```python
from build123d import *

# Parameters (mm, degrees)
BOSS_EXTRUDE1_START = 1
SKETCH2_R           = 17.5
SKETCH2_R_2         = 16.25
SKETCH2_R_3         = 13.75
SKETCH2_R_4         = 12.5
BOSS_EXTRUDE1_DEPTH = 1
FILLET1_R           = 0.5
SKETCH3_R           = 3.75
BOSS_EXTRUDE2_DEPTH = 7.5


with BuildPart() as part:
    # Sketch1 → Revolve1 (revolve)
    with BuildSketch(Plane(origin=(0, 0, 0), x_dir=(1, 0, 0), z_dir=(0, 1, 0)), mode=Mode.PRIVATE) as revolve1_sk:
        Polygon((-36.25, 17.5), (-33.75, 17.5), (-33.75, 5), (33.75, 5), (33.75, 10), (36.25, 10), (36.25, 0), (-36.25, 0), (-46.25, 0), (-46.25, 12.5), align=None)
    revolve(revolve1_sk.sketch.rotate(Axis((-36.25, 0, 0), (1, 0, 0)), 180), axis=Axis((-36.25, 0, 0), (1, 0, 0)))

    # Sketch2 → Boss-Extrude1 (add)
    # profile 1 of 2: a face of its own
    with BuildSketch(Plane(origin=(-33.75, 0, 0), x_dir=(0, 0, -1), z_dir=(1, 0, 0)).offset(BOSS_EXTRUDE1_START)):
        with Locations(Location((0, 0, 0), (0, 0, 180))):
            Circle(SKETCH2_R)
        Circle(SKETCH2_R_2, mode=Mode.SUBTRACT)
    # profile 2 of 2: a face of its own
    with BuildSketch(Plane(origin=(-33.75, 0, 0), x_dir=(0, 0, -1), z_dir=(1, 0, 0)).offset(BOSS_EXTRUDE1_START)):
        with Locations(Location((0, 0, 0), (0, 0, 180))):
            Circle(SKETCH2_R_3)
        Circle(SKETCH2_R_4, mode=Mode.SUBTRACT)
    extrude(amount=-BOSS_EXTRUDE1_DEPTH)

    # Fillet1
    fillet1_edges = [part.edges().sort_by_distance(p)[0] for p in [
        (-32.75, 0, -17.5),
        (-32.75, 0, 12.5),
    ]]
    fillet(fillet1_edges, radius=FILLET1_R)

    # Sketch3 → Boss-Extrude2 (add, symmetric)
    with BuildSketch(Plane(origin=(0, 0, 0), x_dir=(1, 0, 0), z_dir=(0, 1, 0))):
        with BuildLine():
            Line((-46.25, 10), (-46.25, -10))
            Line((-46.25, -10), (-55.85, -7.2))
            ThreePointArc((-55.85, -7.2), (-61.25, 0), (-55.85, 7.2))
            Line((-55.85, 7.2), (-46.25, 10))
        make_face()
        with Locations(Location((-53.75, 0, 0), (0, 0, 270))):
            Circle(SKETCH3_R, mode=Mode.SUBTRACT)
    extrude(amount=BOSS_EXTRUDE2_DEPTH, both=True)


solid = part.part
```
The listing builds one solid part. Answer for the finished solid, in the listing's coordinates (mm). A direction names the side the tool comes from. Give positions to 0.01 mm unless a question says otherwise; leave off trailing zeros. Order: outer loops, then holes, each group sorted by start corner. A loop starts at its lowest first (then second) coordinate and runs counter-clockwise, first axis right, second up. Notation, with made-up numbers: (33, 36.5) - (39, 36.5) arc R21 cw to (39, 50.5) - close; hole circle Ø4 at (2.25, 57). An arc over 180 degrees is marked (long way). Answer in a Markdown table with one row per item. Add a question column.
Q1. The part is cut by section A-A (x = -53.75). Determine the outline of the cut face in (y, z).
Q2. Given P1, Ø2, axis at x = -8, y = -4.5, coming from the -Z side; P2, Ø4.5, axis at x = -54.5, z = -3, coming from the +Y side; P3, Ø5.5, axis at y = 11, z = 3, coming from the -X side, each flat-ended and moving along its own axis, determine where each tip first touches the part or whether it passes through.
Q3. Which of the six approach directions +Z, -Z, +X, -X, +Y, -Y give full straight-line access (tool end or side, diameter ignored) to faces 1 (the flat face through (-33.75, 5.4, -0.2)), 2 (the flat face through (-46.25, 9, 0)), 3 (the flat face through (-46.25, 0, 11)), 4 (the flat face through (-46.25, -9, 0)), 5 (the cylindrical face through (-33.24, 12.2, 6.34))?
Q4. The part is cut by section B-B (x = -25). Determine the outline of the cut face in (y, z), then the cut area to 3 significant figures.
Q5. For a pull along Z with two mould halves and no side action, classify faces 6 (the flat face through (-50, -7.5, 2)), 7 (the flat face through (-50.98, 0.11, 8.62)), 8 (the cylindrical face through (-33.496, 3.755, -11.923)) as released by +Z, released by -Z, zero draft, split by the parting line, or undercut.
Q6. Find the intervals of material crossed by line 1 along Y through (x, z) = (-33.6, 0); line 2 along Y through (x, z) = (-33, 0); line 3 along X through (y, z) = (-9.5, -1), in increasing order. Write a range as [from, to].
Determined:
| question | item | result |
|---|---|---|
| 1 | outline | (-7.5, -7.81) - (7.5, -7.81) - (7.5, -3.75) - (-7.5, -3.75) - close; (-7.5, 3.75) - (7.5, 3.75) - (7.5, 7.81) - (-7.5, 7.81) - close |
| 2 | P1 | stops at z = -3.57 |
| 2 | P2 | stops at y = 7.5 |
| 2 | P3 | stops at x = -46.25 |
| 3 | face 1 | none |
| 3 | face 2 | +Z, -Z, -X, +Y |
| 3 | face 3 | +Z, -X, +Y, -Y |
| 3 | face 4 | +Z, -Z, -X, -Y |
| 3 | face 5 | +X |
| 4 | outline | circle Ø10 at (0, 0) |
| 4 | area | 78.5 mm² |
| 5 | face 6 | zero draft |
| 5 | face 7 | released by +Z |
| 5 | face 8 | undercut |
| 6 | line 1 | y = [-17.5, -16.25], [-13.75, -12.5], [-5, 5], [12.5, 13.75], [16.25, 17.5] |
| 6 | line 2 | y = [-17.43, -16.25], [-13.75, -12.57], [-5, 5], [12.57, 13.75], [16.25, 17.43] |
| 6 | line 3 | x = [-46.25, -33.75], [33.75, 36.25] |
